```python
from build123d import *

# Parameters (mm, degrees)
SKETCH1_W                  = 220
SKETCH1_H                  = 120
BOSS_EXTRUDE1_DEPTH        = 15
CUT_EXTRUDE1_REACH         = 128.194
SKETCH2_W                  = 20.632503002
SKETCH2_H                  = 54.730004003
CUT_EXTRUDE2_REACH         = 128.194
SKETCH3_W                  = 20.25
SKETCH3_H                  = 19.16
SKETCH3_W_2                = 20.5
CUT_EXTRUDE3_REACH         = 128.194
SKETCH4_W                  = 80
SKETCH4_H                  = 14.88
F_6_2_6_2_DIAMETER_HOLE1_D = 6.2
SKETCH8_R                  = 4
CUT_EXTRUDE4_DEPTH         = 0.5
CHAMFER1_SIZE              = 1.8
CHAMFER1_SIZE_2            = 1.039230485


with BuildPart() as part:
    # Sketch1 → Boss-Extrude1 (new body)
    with BuildSketch(Plane(origin=(0, 0, 0), x_dir=(1, 0, 0), z_dir=(0, 1, 0))):
        Rectangle(SKETCH1_W, SKETCH1_H)
    extrude(amount=-BOSS_EXTRUDE1_DEPTH)

    # Sketch2 → Cut-Extrude1 (cut, up to next)
    with BuildSketch(Plane(origin=(0, 0, 0), x_dir=(1, 0, 0), z_dir=(0, 1, 0)), mode=Mode.PRIVATE) as cut_extrude1_sk1:
        with Locations((-99.683748499, 32.634997999)):
            Rectangle(SKETCH2_W, SKETCH2_H)
    cut_extrude1_tool1 = extrude(cut_extrude1_sk1.sketch, amount=-CUT_EXTRUDE1_REACH, mode=Mode.PRIVATE) & part.part
    add(cut_extrude1_tool1.solids().sort_by_distance((-99.683748, 0, -32.634998))[0], mode=Mode.SUBTRACT)

    # Sketch3 → Cut-Extrude2 (cut, up to next)
    with BuildSketch(Plane(origin=(0, 0, 0), x_dir=(1, 0, 0), z_dir=(0, 1, 0)), mode=Mode.PRIVATE) as cut_extrude2_sk1:
        with Locations((-9.875, 18.86)):
            Rectangle(SKETCH3_W, SKETCH3_H)
    cut_extrude2_tool1 = extrude(cut_extrude2_sk1.sketch, amount=-CUT_EXTRUDE2_REACH, mode=Mode.PRIVATE) & part.part
    # Sketch3 → Cut-Extrude2 (cut, up to next)
    with BuildSketch(Plane(origin=(0, 0, 0), x_dir=(1, 0, 0), z_dir=(0, 1, 0)), mode=Mode.PRIVATE) as cut_extrude2_sk2:
        with Locations((30, 18.86)):
            Rectangle(SKETCH3_W_2, SKETCH3_H)
    cut_extrude2_tool2 = extrude(cut_extrude2_sk2.sketch, amount=-CUT_EXTRUDE2_REACH, mode=Mode.PRIVATE) & part.part
    add(cut_extrude2_tool1.solids().sort_by_distance((-9.875, 0, -18.86))[0], mode=Mode.SUBTRACT)
    add(cut_extrude2_tool2.solids().sort_by_distance((30, 0, -18.86))[0], mode=Mode.SUBTRACT)

    # Sketch4 → Cut-Extrude3 (cut, up to next)
    with BuildSketch(Plane(origin=(0, 0, 0), x_dir=(1, 0, 0), z_dir=(0, 1, 0)), mode=Mode.PRIVATE) as cut_extrude3_sk1:
        with Locations((20, -32.16)):
            Rectangle(SKETCH4_W, SKETCH4_H)
    cut_extrude3_tool1 = extrude(cut_extrude3_sk1.sketch, amount=-CUT_EXTRUDE3_REACH, mode=Mode.PRIVATE) & part.part
    add(cut_extrude3_tool1.solids().sort_by_distance((20, 0, 32.16))[0], mode=Mode.SUBTRACT)

    # Ø6.2 (6.2) Diameter Hole1 (through all)
    with Locations(Plane(origin=(0, 0, 0), x_dir=(1, 0, 0), z_dir=(0, 1, 0))):
        with Locations((-30, 0.28), (-50, -14.72), (-70, 0.28), (-90, -14.72)):
            Hole(F_6_2_6_2_DIAMETER_HOLE1_D / 2)

    # Sketch8 → Cut-Extrude4 (cut)
    with BuildSketch(Plane(origin=(0, 0, 0), x_dir=(1, 0, 0), z_dir=(0, 1, 0))):
        with Locations(Location((-90, -14.72, 0), (0, 0, 270))):
            Circle(SKETCH8_R)
        with Locations(Location((-70, 0.28, 0), (0, 0, 270))):
            Circle(SKETCH8_R)
        with Locations(Location((-50, -14.72, 0), (0, 0, 270))):
            Circle(SKETCH8_R)
        with Locations(Location((-30, 0.28, 0), (0, 0, 270))):
            Circle(SKETCH8_R)
    extrude(amount=-CUT_EXTRUDE4_DEPTH, mode=Mode.SUBTRACT)

    # Chamfer1
    # the kernel refuses this chamfer: 1.8, 1.039230485 mm, written as the material it takes off along each edge
    with BuildSketch(Plane(origin=(-90, -0.5, 14.72), x_dir=(-1, 0, 0), z_dir=(0, 0, 1))) as chamfer1_piece_1_section:
        Polygon((3.1, CHAMFER1_SIZE), (3.1 + CHAMFER1_SIZE_2, 0), (3.1, 0), align=None)
    chamfer1_piece_1 = revolve(axis=Axis((-90, -0.5, 14.72), (0, -1, 0)), mode=Mode.PRIVATE)
    chamfer1_piece_1 = chamfer1_piece_1 & Plane(origin=(-90, -1.537716701, 14.72), x_dir=(0, 0, 1), z_dir=(0, 1, 0)) * Cylinder(4, 17, mode=Mode.PRIVATE)
    add(chamfer1_piece_1, mode=Mode.SUBTRACT)
    with BuildSketch(Plane(origin=(-30, -0.5, -0.28), x_dir=(-1, 0, 0), z_dir=(0, 0, 1))) as chamfer1_piece_2_section:
        Polygon((3.1, CHAMFER1_SIZE), (3.1 + CHAMFER1_SIZE_2, 0), (3.1, 0), align=None)
    chamfer1_piece_2 = revolve(axis=Axis((-30, -0.5, -0.28), (0, -1, 0)), mode=Mode.PRIVATE)
    chamfer1_piece_2 = chamfer1_piece_2 & Plane(origin=(-30, -1.537716701, -0.28), x_dir=(0, 0, 1), z_dir=(0, 1, 0)) * Cylinder(4, 17, mode=Mode.PRIVATE)
    add(chamfer1_piece_2, mode=Mode.SUBTRACT)
    with BuildSketch(Plane(origin=(-50, -0.5, 14.72), x_dir=(-1, 0, 0), z_dir=(0, 0, 1))) as chamfer1_piece_3_section:
        Polygon((3.1, CHAMFER1_SIZE), (3.1 + CHAMFER1_SIZE_2, 0), (3.1, 0), align=None)
    chamfer1_piece_3 = revolve(axis=Axis((-50, -0.5, 14.72), (0, -1, 0)), mode=Mode.PRIVATE)
    chamfer1_piece_3 = chamfer1_piece_3 & Plane(origin=(-50, -1.537716701, 14.72), x_dir=(0, 0, 1), z_dir=(0, 1, 0)) * Cylinder(4, 17, mode=Mode.PRIVATE)
    add(chamfer1_piece_3, mode=Mode.SUBTRACT)
    with BuildSketch(Plane(origin=(-70, -0.5, -0.28), x_dir=(-1, 0, 0), z_dir=(0, 0, 1))) as chamfer1_piece_4_section:
        Polygon((3.1, CHAMFER1_SIZE), (3.1 + CHAMFER1_SIZE_2, 0), (3.1, 0), align=None)
    chamfer1_piece_4 = revolve(axis=Axis((-70, -0.5, -0.28), (0, -1, 0)), mode=Mode.PRIVATE)
    chamfer1_piece_4 = chamfer1_piece_4 & Plane(origin=(-70, -1.537716701, -0.28), x_dir=(0, 0, 1), z_dir=(0, 1, 0)) * Cylinder(4, 17, mode=Mode.PRIVATE)
    add(chamfer1_piece_4, mode=Mode.SUBTRACT)


solid = part.part
```
Geometry check sheet. Reference: the model listing, model coordinates, mm. A direction names the side the tool comes from. Coordinates: 2 decimals unless noted, no trailing zeros. Loops run counter-clockwise (first coordinate to the right, second up) from the corner with the lowest first, then second, coordinate; pieces in that order, holes last. Notation, with made-up numbers: (67.25, 81.5) -> (99.25, 81.5) arc R19 cw to (99.25, 104.5) -> close; hole circle Ø6 at (38, 9.25). An arc over 180 degrees is marked (long way). Put each result on its own line as item: value.
1) Tool access check on faces 4 (the flat face through (60, -7, 32)), 5 (the cylindrical face through (-52.434, -0.365, 11.546)), 6 (the flat face through (-110, -7, 28)). Record the directions out of +Z, -Z, +X, -X, +Y, -Y that give a thin tool (end or side, any length) a straight path to the whole face; none if there is none.
Result set:
face 4: +Y, -Y
face 5: +Y
face 6: +Z, -Z, -X, +Y, -Y
2) Cross-section at D-D on z = -0.28. Record the boundary of the cut face in (x, y).
Result set:
outline: (-110, -15) -> (-73.1, -15) -> (-73.1, -2.3) -> (-74, -0.74) -> (-74, 0) -> (-110, 0) -> close; (-66.9, -15) -> (-33.1, -15) -> (-33.1, -2.3) -> (-34, -0.74) -> (-34, 0) -> (-66, 0) -> (-66, -0.74) -> (-66.9, -2.3) -> close; (-26.9, -15) -> (110, -15) -> (110, 0) -> (-26, 0) -> (-26, -0.74) -> (-26.9, -2.3) -> close
3) Cross-section at C-C on y = -8.25. Record the boundary of the cut face in (x, z), plus the area to 3 significant figures.
Result set:
outline: (-110, -5.27) -> (-89.37, -5.27) -> (-89.37, -60) -> (110, -60) -> (110, 60) -> (-110, 60) -> close; hole circle Ø6.2 at (-90, 14.72); hole circle Ø6.2 at (-70, -0.28); hole circle Ø6.2 at (-50, 14.72); hole circle Ø6.2 at (-30, -0.28); hole (-20, -28.44) -> (0.25, -28.44) -> (0.25, -9.28) -> (-20, -9.28) -> close; hole (-20, 24.72) -> (60, 24.72) -> (60, 39.6) -> (-20, 39.6) -> close; hole (19.75, -28.44) -> (40.25, -28.44) -> (40.25, -9.28) -> (19.75, -9.28) -> close
area: 23,200 mm^2
4) Gauge pin test, flat ends, axial feed: pin 1 Ø7 at (x, z) = (-50, 14.72) entering from +Y; pin 2 Ø5 at (y, z) = (-12, -34) entering from -X. Record the tip position at first contact, or that the pin passes through.
Result set:
pin 1: stops at y = -1.61
pin 2: stops at x = -89.37
5) Release check for a two-part mould opening along X. For faces 1 (the flat face through (-20, -7, -19)), 2 (the flat face through (9, -7, -60)), 3 (the flat face through (-89.367, -7, -32)) record: released by +X, released by -X, zero draft, split by the parting line, or undercut.
Result set:
face 1: undercut
face 2: zero draft
face 3: released by -X
6) Cross-section at B-B on z = 34.5. Record the boundary of the cut face in (x, y), plus the area to 3 significant figures.
Result set:
outline: (-110, -15) -> (-20, -15) -> (-20, 0) -> (-110, 0) -> close; (60, -15) -> (110, -15) -> (110, 0) -> (60, 0) -> close
area: 2,100 mm^2
7) Thickness scan on line 1 (X direction, y = -0.3, z = -0.28); line 2 (X direction, y = -11.25, z = -12.5); line 3 (Z direction, x = -30, y = -8.25). Record the ranges inside material, lowest first.
Result set:
line 1: x = -110 to -74, -66 to -34, -26 to 110
line 2: x = -89.37 to -20, 0.25 to 19.75, 40.25 to 110
line 3: z = -60 to -3.38, 2.82 to 60
8) Cross-section at A-A on x = -50. Record the boundary of the cut face in (y, z), plus the area to 3 significant figures.
Result set:
outline: (-15, -60) -> (0, -60) -> (0, 10.72) -> (-0.74, 10.72) -> (-2.3, 11.62) -> (-15, 11.62) -> close; (-15, 17.82) -> (-2.3, 17.82) -> (-0.74, 18.72) -> (0, 18.72) -> (0, 60) -> (-15, 60) -> close
area: 1,700 mm^2
